The model under review builds one solid part; all positions refer to its coordinate system, in mm. Round coordinates to 2 decimals unless told otherwise and drop trailing zeros. Order: outer loops, then holes, each group sorted by start corner. A loop starts at its lowest first (then second) coordinate and runs counter-clockwise, first axis right, second up. Notation, with made-up numbers: M -18.5,25 L -7.5,25 A19 cw -7.5,30 Z; hole C 63,18.5 d10. An arc over 180 degrees is marked long. Use a Markdown table: item, result. Add a question column.
1. Insertion check: P1, Ø5, axis at x = 12, z = -37, coming from the -Y side; P2, Ø5, axis at x = 14.66, z = -36.51, coming from the -Y side; P3, Ø1, axis at y = -41, z = -3.5, coming from the -X side; P4, Ø1.5, axis at y = -41, z = 34, coming from the -X side. Each pin has a flat end and moves straight along its axis. Give the tip position at first contact, or say it passes through.
2. The part is to be moulded in two halves that separate along X. For faces 1 (the conical face through (14.14, -41.68, -38.17)), 2 (the cylindrical face through (46.03, -41.89, -14.5)), say which applies: +X half, -X half, draft (parallel to the pull), parting line (faces both ways), or undercut.
3. Consider section A-A on x = 25. State the section outline as (y, z) points.
4. To check wall thickness, follow probe 1 along Z at (x, y) = (3.5, -40.95); probe 2 along X at (y, z) = (-42.9, 1); probe 3 along Z at (x, y) = (-2.5, -42.05). State the ranges of each line that lie inside material, in increasing order.
5. Consider section B-B on z = 18.5. State the section outline as (x, y) points, then the cut area to 3 significant figures.
from build123d import *

# Parameters (mm, degrees)
SKETCH3_R                                      = 48.26
SKETCH3_R_2                                    = 34.925
BOSS_EXTRUDE1_DEPTH                            = 3.1496
CSK_FOR_M4_FLAT_HEAD_MACHINE_SCREW2_AT_2_COUNT = 2
CSK_FOR_M4_FLAT_HEAD_MACHINE_SCREW2_AT_2_PITCH = 61.784162113
CSK_FOR_M4_FLAT_HEAD_MACHINE_SCREW2_AT_3_COUNT = 2
CSK_FOR_M4_FLAT_HEAD_MACHINE_SCREW2_AT_3_PITCH = 87.376
CSK_FOR_M4_FLAT_HEAD_MACHINE_SCREW2_AT_4_COUNT = 2
CSK_FOR_M4_FLAT_HEAD_MACHINE_SCREW2_AT_4_PITCH = 61.784162113
CSK_FOR_4_FLAT_HEAD_MACHINE_SCREW1_AT_2_COUNT  = 2
CSK_FOR_4_FLAT_HEAD_MACHINE_SCREW1_AT_2_PITCH  = 19.05
CSK_FOR_4_FLAT_HEAD_MACHINE_SCREW1_AT_3_COUNT  = 2
CSK_FOR_4_FLAT_HEAD_MACHINE_SCREW1_AT_3_PITCH  = 35.79885845
CSK_FOR_4_FLAT_HEAD_MACHINE_SCREW1_AT_4_COUNT  = 2
CSK_FOR_4_FLAT_HEAD_MACHINE_SCREW1_AT_4_PITCH  = 51.698767879
CSK_FOR_4_FLAT_HEAD_MACHINE_SCREW1_AT_5_COUNT  = 2
CSK_FOR_4_FLAT_HEAD_MACHINE_SCREW1_AT_5_PITCH  = 63.760255082
CSK_FOR_4_FLAT_HEAD_MACHINE_SCREW1_AT_6_COUNT  = 2
CSK_FOR_4_FLAT_HEAD_MACHINE_SCREW1_AT_6_PITCH  = 73.02909889


with BuildPart() as part:
    # Sketch3 → Boss-Extrude1 (new body)
    with BuildSketch(Plane(origin=(0, -40.33266, 0), x_dir=(1, 0, 0), z_dir=(0, 1, 0))):
        Circle(SKETCH3_R)
        Circle(SKETCH3_R_2, mode=Mode.SUBTRACT)
    extrude(amount=-BOSS_EXTRUDE1_DEPTH)

    # Sketch18 → CSK for M4 Flat Head Machine Screw2 (revolve, cut)
    with BuildSketch(Plane(origin=(0, -40.33266, 43.688), x_dir=(0, 0, 1), z_dir=(1, 0, 0))):
        Polygon((0, 0), (0, 3.1496), (2.25, 3.1496), (2.25, 2.35), (4.6, 0), align=None)
    csk_for_m4_flat_head_machine_screw2 = revolve(axis=Axis((0, -33.98266, 43.688), (0, -1, 0)), mode=Mode.SUBTRACT)

    # CSK for M4 Flat Head Machine Screw2 at 2: CSK for M4 Flat Head Machine Screw2 ×2
    with Locations(*[Vector(0.707106781, 0, -0.707106781) * (i * CSK_FOR_M4_FLAT_HEAD_MACHINE_SCREW2_AT_2_PITCH) for i in range(1, CSK_FOR_M4_FLAT_HEAD_MACHINE_SCREW2_AT_2_COUNT)]):
        add(csk_for_m4_flat_head_machine_screw2, mode=Mode.SUBTRACT)

    # CSK for M4 Flat Head Machine Screw2 at 3: CSK for M4 Flat Head Machine Screw2 ×2
    with Locations(*[(0, 0, -i * CSK_FOR_M4_FLAT_HEAD_MACHINE_SCREW2_AT_3_PITCH) for i in range(1, CSK_FOR_M4_FLAT_HEAD_MACHINE_SCREW2_AT_3_COUNT)]):
        add(csk_for_m4_flat_head_machine_screw2, mode=Mode.SUBTRACT)

    # CSK for M4 Flat Head Machine Screw2 at 4: CSK for M4 Flat Head Machine Screw2 ×2
    with Locations(*[Vector(-0.707106781, 0, -0.707106781) * (i * CSK_FOR_M4_FLAT_HEAD_MACHINE_SCREW2_AT_4_PITCH) for i in range(1, CSK_FOR_M4_FLAT_HEAD_MACHINE_SCREW2_AT_4_COUNT)]):
        add(csk_for_m4_flat_head_machine_screw2, mode=Mode.SUBTRACT)

    # Sketch9 → CSK for #4 Flat Head Machine Screw1 (revolve, cut)
    with BuildSketch(Plane(origin=(14.657877005, -43.48226, 36.514549445), x_dir=(0, 0, -1), z_dir=(1, 0, 0))):
        Polygon((0, 0), (0, 3.1496), (1.63195, 3.1496), (1.63195, 1.921172758), (3.302, 0), align=None)
    csk_for_4_flat_head_machine_screw1 = revolve(axis=Axis((14.657877005, -49.83226, 36.514549445), (0, 1, 0)), mode=Mode.SUBTRACT)

    # CSK for #4 Flat Head Machine Screw1 at 2: CSK for #4 Flat Head Machine Screw1 ×2
    with Locations(*[Vector(0.810235621, 0, -0.58610429) * (i * CSK_FOR_4_FLAT_HEAD_MACHINE_SCREW1_AT_2_PITCH) for i in range(1, CSK_FOR_4_FLAT_HEAD_MACHINE_SCREW1_AT_2_COUNT)]):
        add(csk_for_4_flat_head_machine_screw1, mode=Mode.SUBTRACT)

    # CSK for #4 Flat Head Machine Screw1 at 3: CSK for #4 Flat Head Machine Screw1 ×2
    with Locations(*[Vector(0.65696386, 0, -0.753922069) * (i * CSK_FOR_4_FLAT_HEAD_MACHINE_SCREW1_AT_3_PITCH) for i in range(1, CSK_FOR_4_FLAT_HEAD_MACHINE_SCREW1_AT_3_COUNT)]):
        add(csk_for_4_flat_head_machine_screw1, mode=Mode.SUBTRACT)

    # CSK for #4 Flat Head Machine Screw1 at 4: CSK for #4 Flat Head Machine Screw1 ×2
    with Locations(*[Vector(0.454915217, 0, -0.890534752) * (i * CSK_FOR_4_FLAT_HEAD_MACHINE_SCREW1_AT_4_PITCH) for i in range(1, CSK_FOR_4_FLAT_HEAD_MACHINE_SCREW1_AT_4_COUNT)]):
        add(csk_for_4_flat_head_machine_screw1, mode=Mode.SUBTRACT)

    # CSK for #4 Flat Head Machine Screw1 at 5: CSK for #4 Flat Head Machine Screw1 ×2
    with Locations(*[Vector(0.242078526, 0, -0.97025666) * (i * CSK_FOR_4_FLAT_HEAD_MACHINE_SCREW1_AT_5_PITCH) for i in range(1, CSK_FOR_4_FLAT_HEAD_MACHINE_SCREW1_AT_5_COUNT)]):
        add(csk_for_4_flat_head_machine_screw1, mode=Mode.SUBTRACT)

    # CSK for #4 Flat Head Machine Screw1 at 6: CSK for #4 Flat Head Machine Screw1 ×2
    with Locations(*[(0, 0, -i * CSK_FOR_4_FLAT_HEAD_MACHINE_SCREW1_AT_6_PITCH) for i in range(1, CSK_FOR_4_FLAT_HEAD_MACHINE_SCREW1_AT_6_COUNT)]):
        add(csk_for_4_flat_head_machine_screw1, mode=Mode.SUBTRACT)


solid = part.part
Answer block:
| question | item | result |
|---|---|---|
| 1 | P1 | y = -43.48 |
| 1 | P2 | y = -42.57 |
| 1 | P3 | x = -48.17 |
| 1 | P4 | x = -34.98 |
| 2 | face 1 | undercut |
| 2 | face 2 | parting line |
| 3 | outline | M -43.48,-41.28 L -40.33,-41.28 L -40.33,-24.39 L -43.48,-24.39 Z; M -43.48,24.39 L -40.33,24.39 L -40.33,41.28 L -43.48,41.28 Z |
| 4 | probe 1 | -48.13 to -45.59, -41.79 to -34.75, 34.75 to 41.79, 45.59 to 48.13 |
| 4 | probe 2 | -48.25 to -45.7, -41.67 to -34.91, 34.91 to 41.67, 45.7 to 48.25 |
| 4 | probe 3 | -48.2 to -45.12, -42.25 to -34.84, 34.84 to 42.25, 45.12 to 48.2 |
| 5 | outline | M -44.57,-43.48 L -29.62,-43.48 L -29.62,-40.33 L -44.57,-40.33 Z; M 29.62,-43.48 L 44.57,-43.48 L 44.57,-40.33 L 29.62,-40.33 Z |
| 5 | area | 94.2 mm^2 |
